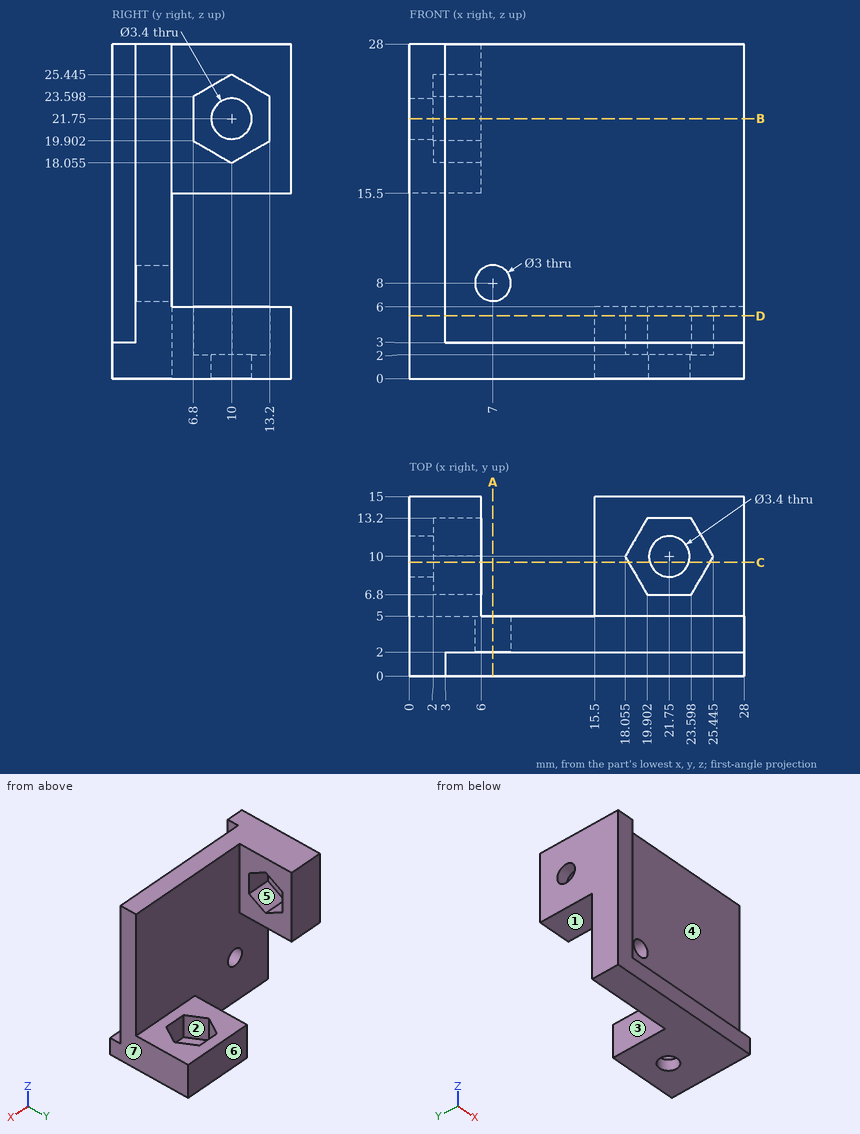
Here's the drawing with two shaded views (mm, measured from the low corner). I have some questions. A direction names the side the tool comes from. Give positions to 0.01 mm unless a question says otherwise; leave off trailing zeros. Order: outer loops, then holes, each group sorted by start corner. A loop starts at its lowest first (then second) coordinate and runs counter-clockwise, first axis right, second up. Notation, with made-up numbers: (-21, 5.25) -> (24, 5.25) arc R23 ccw to (24, 40.25) -> close; hole circle Ø9 at (37.5, 9.25). An arc over 180 degrees is marked (long way). One line per item, written item: value. Start each with the question number.
1. Imagine slicing it at C-C, the plane y = 9.5. List the corners of the cut face in (x, z) for me (1 decimal).
2. Imagine slicing it at A-A, the plane x = 7. List the corners of the cut face in (y, z) for me.
3. I need wall thicknesses on probe 1 along Z at (x, y) = (7, 2.8); probe 2 along Y at (x, z) = (21.75, 1.5); probe 3 along Y at (x, z) = (16.25, 4.5). Which ranges of each line are inside material? Lowest first, please. Write a range as from..to.
4. Imagine slicing it at B-B, the plane z = 21.75. List the corners of the cut face in (x, y) for me, plus the area to 3 significant figures.
5. We'd pull the mould along Y, two halves only. Please class the marked faces 4, 5, 6 and 7: released by +Y, released by -Y, zero draft, split by the parting line, or undercut.
6. For the marked faces 1, 2 and 3, which set-ups out of +Z, -Z, +X, -X, +Y, -Y let a thin tool reach every point of the face, with its end or its side?
7. Imagine slicing it at D-D, the plane z = 5.25. List the corners of the cut face in (x, y) for me (1 decimal).
8. Will these pins go through, and if not, where does the flat tip stop? pin 1 Ø10 at (x, z) = (24, 7.5) entering from +Y; pin 2 Ø5 at (y, z) = (8.5, 3.5) entering from -X; pin 3 Ø3 at (y, z) = (9, 21.5) entering from +X; pin 4 Ø12.5 at (x, z) = (13.5, 11) entering from -Y.
Values follow:
1. outline: (0, 15.5) -> (6, 15.5) -> (6, 18.3) -> (2, 18.3) -> (2, 20.1) -> (0, 20.1) -> close; (0, 23.4) -> (2, 23.4) -> (2, 25.2) -> (6, 25.2) -> (6, 28) -> (0, 28) -> close; (15.5, 0) -> (20.1, 0) -> (20.1, 2) -> (18.3, 2) -> (18.3, 6) -> (15.5, 6) -> close; (23.4, 0) -> (28, 0) -> (28, 6) -> (25.2, 6) -> (25.2, 2) -> (23.4, 2) -> close
2. outline: (0, 0) -> (5, 0) -> (5, 6.5) -> (2, 6.5) -> (2, 3) -> (0, 3) -> close; (2, 9.5) -> (5, 9.5) -> (5, 28) -> (2, 28) -> close
3. probe 1: z = 0..6.5, 9.5..28
3. probe 2: y = 0..8.3, 11.7..15
3. probe 3: y = 2..15
4. outline: (0, 0) -> (3, 0) -> (3, 2) -> (28, 2) -> (28, 5) -> (6, 5) -> (6, 6.8) -> (2, 6.8) -> (2, 8.3) -> (0, 8.3) -> close; (0, 11.7) -> (2, 11.7) -> (2, 13.2) -> (6, 13.2) -> (6, 15) -> (0, 15) -> close
4. area: 118 mm2
5. face 4: released by -Y
5. face 5: undercut
5. face 6: released by +Y
5. face 7: zero draft
6. face 1: -Z, +X, -X, +Y
6. face 2: +Z
6. face 3: +Z, -Z, -X, +Y
7. outline: (0, 0) -> (3, 0) -> (3, 2) -> (28, 2) -> (28, 15) -> (15.5, 15) -> (15.5, 5) -> (0, 5) -> close; hole (18.1, 10) -> (19.9, 6.8) -> (23.6, 6.8) -> (25.4, 10) -> (23.6, 13.2) -> (19.9, 13.2) -> close
8. pin 1: stops at y = 15
8. pin 2: stops at x = 15.5
8. pin 3: stops at x = 2
8. pin 4: stops at y = 2
